The listing builds one solid part. Answer for the finished solid, in the listing's coordinates (mm). A direction names the side the tool comes from. Give positions to 0.01 mm unless a question says otherwise; leave off trailing zeros. Order: outer loops, then holes, each group sorted by start corner. A loop starts at its lowest first (then second) coordinate and runs counter-clockwise, first axis right, second up. Notation, with made-up numbers: M 22,-2.75 L 61,-2.75 A30 cw 61,26.25 Z; hole C 57.25,-25.5 d11. An arc over 180 degrees is marked long. Answer as a JSON object with one key per item and string values. Group by question number.
```python
from build123d import *

# Parameters (mm, degrees)
ESBO_O1_W                        = 93
ESBO_O1_H                        = 88
RESSALTO_EXTRUS_O2_DEPTH         = 35
ESBO_O1_5_W                      = 93
ESBO_O1_5_H                      = 88
RESSALTO_EXTRUS_O3_DEPTH         = 8
ESBO_O1_7_W                      = 93
ESBO_O1_7_H                      = 88
ESBO_O1_7_R                      = 2
RESSALTO_EXTRUS_O6_DEPTH         = 5
ESBO_O4_R                        = 2.218632056
RESSALTO_EXTRUS_O7_DEPTH         = 3
ESBO_O5_W                        = 88.65
ESBO_O5_H                        = 82.92
RESSALTO_EXTRUS_O8_DEPTH         = 2
ESBO_O7_W                        = 12.6
ESBO_O7_H                        = 15.81
CORTE_EXTRUS_O1_DEPTH            = 146.086181285
ESBO_O8_W                        = 12.6
ESBO_O8_H                        = 15.81
CORTE_EXTRUS_O2_DEPTH            = 146.086181285
FURO_COM_FOLGA_DE_41_D           = 3.2639
FURO_COM_FOLGA_DE_41_DEPTH       = 8
FURO_COM_FOLGA_DE_41_CSINK_D     = 4.5339
FURO_COM_FOLGA_DE_41_CSINK_ANGLE = 90
FURO_COM_FOLGA_DE_41_TIP         = 0.980574487
RESSALTO_EXTRUS_O10_DEPTH        = 2


with BuildPart() as part:
    # Esbo_o1 → Ressalto-extrus_o2 (new body)
    with BuildSketch(Plane(origin=(0, 0, 0), x_dir=(1, 0, 0), z_dir=(0, 1, 0))):
        with BuildLine():
            Line((0, -3), (93, -3))
            ThreePointArc((93, -3), (95.121320344, -2.121320344), (96, 0))
            Line((96, 0), (96, 88))
            ThreePointArc((96, 88), (95.121320344, 90.121320344), (93, 91))
            Line((93, 91), (0, 91))
            ThreePointArc((0, 91), (-2.121320344, 90.121320344), (-3, 88))
            Line((-3, 88), (-3, 0))
            ThreePointArc((-3, 0), (-2.121320344, -2.121320344), (0, -3))
        make_face()
        with Locations((46.5, 44)):
            Rectangle(ESBO_O1_W, ESBO_O1_H, mode=Mode.SUBTRACT)
    extrude(amount=RESSALTO_EXTRUS_O2_DEPTH)

    # Esbo_o1_5 → Ressalto-extrus_o3 (add)
    with BuildSketch(Plane(origin=(0, 0, 0), x_dir=(1, 0, 0), z_dir=(0, 1, 0))):
        with Locations((46.5, 44)):
            Rectangle(ESBO_O1_5_W, ESBO_O1_5_H)
    extrude(amount=RESSALTO_EXTRUS_O3_DEPTH)

    # Esbo_o1_7 → Ressalto-extrus_o6 (add)
    # profile 1 of 3: a face of its own
    with BuildSketch(Plane(origin=(0, 0, 0), x_dir=(1, 0, 0), z_dir=(0, 1, 0))):
        with BuildLine():
            Line((0, -3), (93, -3))
            ThreePointArc((93, -3), (95.121320344, -2.121320344), (96, 0))
            Line((96, 0), (96, 88))
            ThreePointArc((96, 88), (95.121320344, 90.121320344), (93, 91))
            Line((93, 91), (0, 91))
            ThreePointArc((0, 91), (-2.121320344, 90.121320344), (-3, 88))
            Line((-3, 88), (-3, 0))
            ThreePointArc((-3, 0), (-2.121320344, -2.121320344), (0, -3))
        make_face()
        with Locations((46.5, 44)):
            Rectangle(ESBO_O1_7_W, ESBO_O1_7_H, mode=Mode.SUBTRACT)
    # profile 2 of 3: a face of its own
    with BuildSketch(Plane(origin=(0, 0, 0), x_dir=(1, 0, 0), z_dir=(0, 1, 0))):
        with BuildLine():
            Line((-3, 38.5), (-13, 38.5))
            ThreePointArc((-13, 38.5), (-14.414213562, 39.085786438), (-15, 40.5))
            Line((-15, 40.5), (-15, 47.5))
            ThreePointArc((-15, 47.5), (-14.414213562, 48.914213562), (-13, 49.5))
            Line((-13, 49.5), (-3, 49.5))
            Line((-3, 49.5), (-3, 38.5))
        make_face()
        with Locations(Location((-8.5, 44, 0), (0, 0, 270))):
            Circle(ESBO_O1_7_R, mode=Mode.SUBTRACT)
    # profile 3 of 3: a face of its own
    with BuildSketch(Plane(origin=(0, 0, 0), x_dir=(1, 0, 0), z_dir=(0, 1, 0))):
        with BuildLine():
            Line((57, -3), (68, -3))
            Line((68, -3), (68, -13))
            ThreePointArc((68, -13), (67.414213562, -14.414213562), (66, -15))
            Line((66, -15), (59, -15))
            ThreePointArc((59, -15), (57.585786438, -14.414213562), (57, -13))
            Line((57, -13), (57, -3))
        make_face()
        with Locations(Location((62.5, -8.5, 0), (0, 0, 270))):
            Circle(ESBO_O1_7_R, mode=Mode.SUBTRACT)
    extrude(amount=RESSALTO_EXTRUS_O6_DEPTH)

    # Esbo_o4 → Ressalto-extrus_o7 (add)
    # profile 1 of 2: a face of its own
    with BuildSketch(Plane(origin=(0, 35, 0), x_dir=(1, 0, 0), z_dir=(0, 1, 0))):
        with BuildLine():
            Line((41, -3), (52, -3))
            Line((52, -3), (52, -13))
            ThreePointArc((52, -13), (51.414213562, -14.414213562), (50, -15))
            Line((50, -15), (43, -15))
            ThreePointArc((43, -15), (41.585786438, -14.414213562), (41, -13))
            Line((41, -13), (41, -3))
        make_face()
        with Locations(Location((46.5, -8.5, 0), (0, 0, 270))):
            Circle(ESBO_O4_R, mode=Mode.SUBTRACT)
    # profile 2 of 2: a face of its own
    with BuildSketch(Plane(origin=(0, 35, 0), x_dir=(1, 0, 0), z_dir=(0, 1, 0))):
        with BuildLine():
            Line((43, 103), (50, 103))
            ThreePointArc((50, 103), (51.414213562, 102.414213562), (52, 101))
            Line((52, 101), (52, 91))
            Line((52, 91), (41, 91))
            Line((41, 91), (41, 101))
            ThreePointArc((41, 101), (41.585786438, 102.414213562), (43, 103))
        make_face()
        with Locations(Location((46.5, 96.5, 0), (0, 0, 90))):
            Circle(ESBO_O4_R, mode=Mode.SUBTRACT)
    extrude(amount=-RESSALTO_EXTRUS_O7_DEPTH)

    # Esbo_o5 → Ressalto-extrus_o8 (add)
    with BuildSketch(Plane(origin=(0, 8, 0), x_dir=(1, 0, 0), z_dir=(0, 1, 0))):
        with Locations((46.5, 44)):
            Rectangle(ESBO_O5_W, ESBO_O5_H)
    extrude(amount=RESSALTO_EXTRUS_O8_DEPTH)

    # Esbo_o7 → Corte-extrus_o1 (cut, through all)
    with BuildSketch(Plane.XY.offset(-88)):
        with Locations((67.38, 15.905)):
            Rectangle(ESBO_O7_W, ESBO_O7_H)
        with Locations((84.02, 15.905)):
            Rectangle(ESBO_O7_W, ESBO_O7_H)
    extrude(amount=-CORTE_EXTRUS_O1_DEPTH, mode=Mode.SUBTRACT)

    # Esbo_o8 → Corte-extrus_o2 (cut, through all)
    with BuildSketch(Plane(origin=(0, 0, 0), x_dir=(-1, 0, 0), z_dir=(0, 0, -1))):
        with Locations((-76.29, 15.905)):
            Rectangle(ESBO_O8_W, ESBO_O8_H)
    extrude(amount=-CORTE_EXTRUS_O2_DEPTH, mode=Mode.SUBTRACT)

    # Furo com folga de _41
    with Locations(Plane(origin=(6.12, 10, -82.28), x_dir=(0, 0, 1), z_dir=(0, 1, 0))):
        with Locations((0, 0), (76.45, 0), (76.45, 80.77)):
            CounterSinkHole(FURO_COM_FOLGA_DE_41_D / 2, FURO_COM_FOLGA_DE_41_CSINK_D / 2, depth=FURO_COM_FOLGA_DE_41_DEPTH, counter_sink_angle=FURO_COM_FOLGA_DE_41_CSINK_ANGLE)
            with Locations((0, 0, -(FURO_COM_FOLGA_DE_41_DEPTH + FURO_COM_FOLGA_DE_41_TIP / 2))):  # 118° drill point
                Cone(0, FURO_COM_FOLGA_DE_41_D / 2, FURO_COM_FOLGA_DE_41_TIP, mode=Mode.SUBTRACT)

    # Esbo_o14 → Ressalto-extrus_o10 (add)
    with BuildSketch(Plane(origin=(0, 35, 0), x_dir=(1, 0, 0), z_dir=(0, 1, 0))):
        with BuildLine():
            Line((1.5, 89.5), (91.5, 89.5))
            ThreePointArc((91.5, 89.5), (93.621320344, 88.621320344), (94.5, 86.5))
            Line((94.5, 86.5), (94.5, 1.5))
            ThreePointArc((94.5, 1.5), (93.621320344, -0.621320344), (91.5, -1.5))
            Line((91.5, -1.5), (1.5, -1.5))
            ThreePointArc((1.5, -1.5), (-0.621320344, -0.621320344), (-1.5, 1.5))
            Line((-1.5, 1.5), (-1.5, 86.5))
            ThreePointArc((-1.5, 86.5), (-0.621320344, 88.621320344), (1.5, 89.5))
        make_face()
        with BuildLine():
            Line((3.5, 87.5), (89.5, 87.5))
            ThreePointArc((89.5, 87.5), (91.621320344, 86.621320344), (92.5, 84.5))
            Line((92.5, 84.5), (92.5, 3.5))
            ThreePointArc((92.5, 3.5), (91.621320344, 1.378679656), (89.5, 0.5))
            Line((89.5, 0.5), (3.5, 0.5))
            ThreePointArc((3.5, 0.5), (1.378679656, 1.378679656), (0.5, 3.5))
            Line((0.5, 3.5), (0.5, 84.5))
            ThreePointArc((0.5, 84.5), (1.378679656, 86.621320344), (3.5, 87.5))
        make_face(mode=Mode.SUBTRACT)
    extrude(amount=RESSALTO_EXTRUS_O10_DEPTH)


solid = part.part
```
Item 1: Determine the mould class of faces 1 (the cylindrical face through (1.4, 35.99, -1.36)), 2 (the flat face through (46, 17, 3)), 3 (the cylindrical face through (-0.64, 35.99, -88.6)) for opening direction X: released by +X, released by -X, zero draft, split by the parting line, or undercut.
Item 2: Section A-A (z = -96.5) is taken. Determine the outline of the cut face in (x, y), and give its area (3 significant figures).
Item 3: Section D-D (x = 33) is taken. Determine the outline of the cut face in (y, z).
Item 4: Section B-B (x = 46.5) is taken. Count the separate pieces of the cut face and the enclosed holes in it, and give its area (3 significant figures).
Item 5: Flat-ended cylindrical pins translate along their axes: P1, Ø4.5, axis at x = 62.5, z = 8.5, coming from the +Y side; P2, Ø3.5, axis at x = 66, z = -89.5, coming from the -Y side; P3, Ø21.5, axis at y = 25, z = -47, coming from the -X side; P4, Ø5.5, axis at x = 44.5, z = 9, coming from the -Y side. Find the tip coordinate at first contact, or state that the pin passes through.
Item 6: Section C-C (y = 16.5) is taken. Determine the outline of the cut face in (x, z).
Item 7: A tool of negligible diameter and unlimited length cuts with its end or side. For faces 4 (the flat face through (52, 34, 8)), 5 (the cylindrical face through (91.6, 35.99, -86.64)), 6 (the flat face through (-8, 2, -38.5)), 7 (the cylindrical face through (-7.148, 2.465, -45.474)), from which of +Z, -Z, +X, -X, +Y, -Y can it reach the whole face along a straight path? Write none if from no direction.
Item 8: Consider probe 1 along X at (y, z) = (8.5, -61) (3 decimals); probe 2 along X at (y, z) = (4.5, -5.83); probe 3 along Z at (x, y) = (86.89, 5.25). Determine where each line is inside the solid, lowest interval first. Write a range as from..to.
Values found:
{
 "1": {"face 1": "undercut", "face 2": "zero draft", "face 3": "released by -X"},
 "2": {"outline": "M 41,32 L 44.28,32 L 44.28,35 L 41,35 Z; M 48.72,32 L 52,32 L 52,35 L 48.72,35 Z", "area": "19.7 mm^2"},
 "3": {"outline": "M 0,-91 L 35,-91 L 35,-89.5 L 37,-89.5 L 37,-87.5 L 35,-87.5 L 35,-88 L 8,-88 L 8,-85.46 L 10,-85.46 L 10,-2.54 L 8,-2.54 L 8,0 L 35,0 L 35,-0.5 L 37,-0.5 L 37,1.5 L 35,1.5 L 35,3 L 0,3 Z"},
 "4": {"separate pieces": "3", "enclosed holes": "0", "area": "1,130 mm^2"},
 "5": {"P1": "stops at y = 5", "P2": "stops at y = 0", "P3": "stops at x = -3", "P4": "stops at y = 32"},
 "6": {"outline": "M -3,-88 A3 ccw 0,-91 L 61.08,-91 L 61.08,-88 L 0,-88 L 0,0 L 69.99,0 L 69.99,3 L 0,3 A3 ccw -3,0 Z; M 73.68,-91 L 77.72,-91 L 77.72,-88 L 73.68,-88 Z; M 82.59,0 L 93,0 L 93,-88 L 90.32,-88 L 90.32,-91 L 93,-91 A3 ccw 96,-88 L 96,0 A3 ccw 93,3 L 82.59,3 Z"},
 "7": {"face 4": "+Z, +X, +Y, -Y", "face 5": "+Y", "face 6": "+Z, -X, +Y, -Y", "face 7": "+Y, -Y"},
 "8": {"probe 1": "x = -3..0, 2.175..90.825, 93..96", "probe 2": "x = -3..4.49, 7.75..85.26, 88.52..96", "probe 3": "z = -91..-7.46, -4.2..3"}
}
